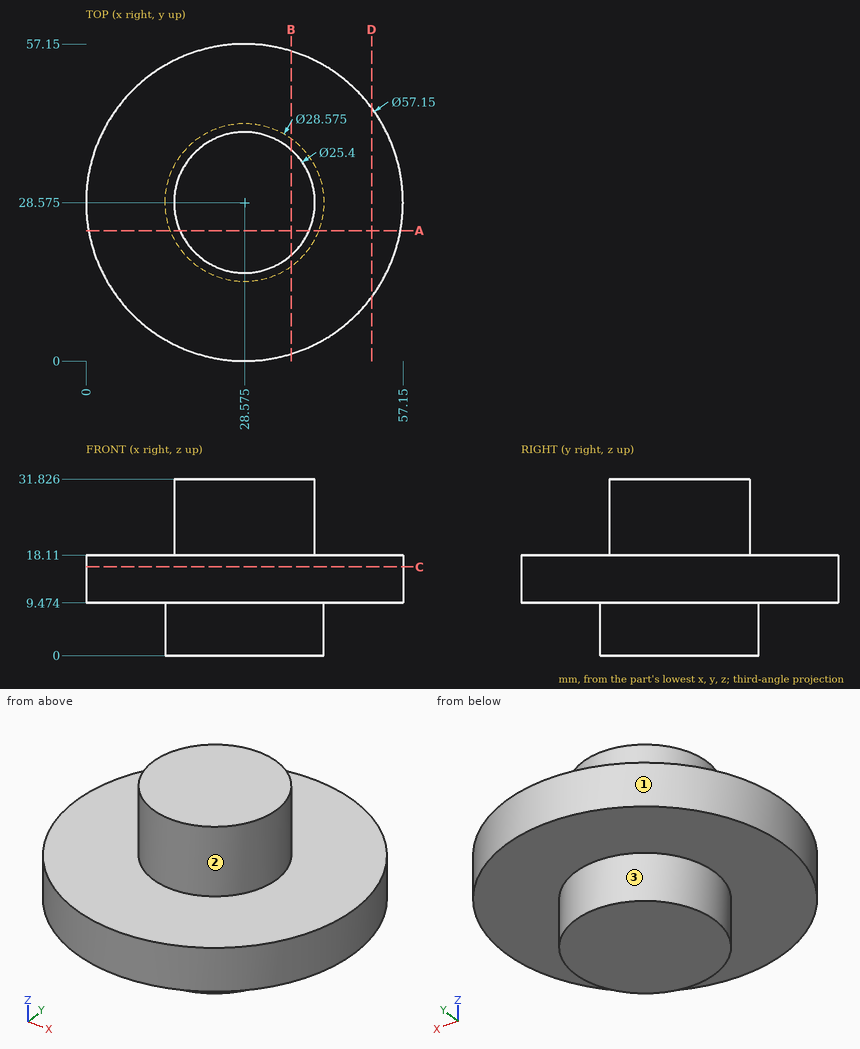
Design review of the part shown in the three views and the two pictorial views. Dimensions are in mm from the part's minimum x, y and z. A direction names the side the tool comes from. Give positions to 0.01 mm unless a question says otherwise; leave off trailing zeros. Loops run counter-clockwise (first coordinate to the right, second up) from the corner with the lowest first, then second, coordinate; pieces in that order, holes last. Notation, with made-up numbers: M 26,-3.75 L 43,-3.75 A26 cw 43,12.25 Z; hole C 4.25,5.25 d7. An arc over 180 degrees is marked long. Put each result on its own line as item: value. Start each with the question number.
(1) Wall thickness on L1, parallel to Z at x = 42, y = 40.5; L2, parallel to Z at x = 25, y = 42; L3, parallel to Y at x = 28, z = 8.5: over which ranges is each line inside the solid? List them lowest first.
(2) For pin 1 (1 mm diameter, centred on x = 36.5, z = 24, fed in from +Y); pin 2 (1.5 mm diameter, centred on y = 34.5, z = 12.5, fed in from -X); pin 3 (8 mm diameter, centred on y = 40, z = 6, fed in from -X) (1 decimal), all flat-tipped, find the tip position at first contact; note any pin that passes through.
(3) Add section D-D, the plane x = 51.5. Write out the cut boundary in (y, z), then the cut area to 3 significant figures.
(4) Add section C-C, the plane z = 16. Write out the cut boundary in (x, y) (3 decimals), then the cut area to 3 significant figures.
(5) Add section B-B, the plane x = 37. Write out the cut boundary in (y, z).
(6) Add section A-A, the plane y = 23.5. Write out the cut boundary in (x, z), then the cut area to 3 significant figures.
(7) Machinability: for the marked faces 1, 2 and 3, which of the approach directions +Z, -Z, +X, -X, +Y, -Y give a long, thin tool a straight path to every point of the face, cutting with its end or side? Answer none if there is none.
Result:
1. L1: z = 9.47 to 18.11
1. L2: z = 0 to 18.11
1. L3: y = 14.3 to 42.85
2. pin 1: stops at y = 38.88
2. pin 2: stops at x = 0.47
2. pin 3: stops at x = 1.6
3. outline: M 11.52,9.47 L 45.63,9.47 L 45.63,18.11 L 11.52,18.11 Z
3. area: 295 mm^2
4. outline: C 28.575,28.575 d57.15
4. area: 2,570 mm^2
5. outline: M 1.27,9.47 L 17.04,9.47 L 17.04,0 L 40.11,0 L 40.11,9.47 L 55.88,9.47 L 55.88,18.11 L 38.08,18.11 L 38.08,31.83 L 19.07,31.83 L 19.07,18.11 L 1.27,18.11 Z
6. outline: M 0.45,9.47 L 15.22,9.47 L 15.22,0 L 41.93,0 L 41.93,9.47 L 56.7,9.47 L 56.7,18.11 L 40.22,18.11 L 40.22,31.83 L 16.93,31.83 L 16.93,18.11 L 0.45,18.11 Z
6. area: 1,060 mm^2
7. face 1: +Z, -Z
7. face 2: +Z
7. face 3: -Z
